CAD build for the part. Positions are in the model's coordinates, mm. Face numbers are marked on the shaded views. A direction names the side the tool comes from. Give positions to 0.01 mm unless a question says otherwise; leave off trailing zeros. Loops run counter-clockwise (first coordinate to the right, second up) from the corner with the lowest first, then second, coordinate; pieces in that order, holes last.
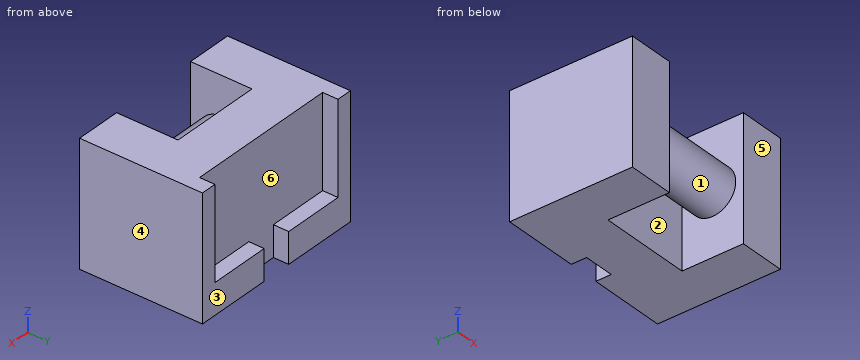
```python
from build123d import *

# Parameters (mm, degrees)
SKETCH2_W           = 76.2
SKETCH2_H           = 25.4
BOSS_EXTRUDE1_DEPTH = 50.8
SKETCH3_W           = 19.05
SKETCH3_H           = 50.8
BOSS_EXTRUDE2_DEPTH = 25.4
SKETCH4_R           = 9.525
BOSS_EXTRUDE3_DEPTH = 50.8
SKETCH7_W           = 12.6492
SKETCH7_H           = 12.7254
CUT_EXTRUDE1_DEPTH  = 6.35


with BuildPart() as part:
    # Sketch2 → Boss-Extrude1 (new body)
    with BuildSketch(Plane.XY):
        with Locations((30.119125683, -4.19863388)):
            Rectangle(SKETCH2_W, SKETCH2_H)
    extrude(amount=BOSS_EXTRUDE1_DEPTH)

    # Sketch3 → Boss-Extrude2 (add)
    with BuildSketch(Plane.XZ.offset(16.89863388)):
        with Locations((1.544125683, 25.4)):
            Rectangle(SKETCH3_W, SKETCH3_H)
        with Locations((58.694125683, 25.4)):
            Rectangle(SKETCH3_W, SKETCH3_H)
    extrude(amount=BOSS_EXTRUDE2_DEPTH)

    # Sketch4 → Boss-Extrude3 (add)
    with BuildSketch(Plane(origin=(11.069125683, 0, 0), x_dir=(0, 0, -1), z_dir=(1, 0, 0))):
        with Locations(Location((-25.4, -29.59863388, 0), (0, 0, 180))):
            Circle(SKETCH4_R)
    extrude(amount=BOSS_EXTRUDE3_DEPTH)

    # Sketch7 → Cut-Extrude1 (cut)
    with BuildSketch(Plane(origin=(0, 8.50136612, 0), x_dir=(1, 0, 0), z_dir=(0, 1, 0))):
        Polygon((-1.610554317, -12.7254), (-1.610554317, -50.8), (61.798005683, -50.8), (61.798005683, -12.7254), (36.418325683, -12.7254), (23.769125683, -12.7254), align=None)
        with Locations((30.093725683, -6.3627)):
            Rectangle(SKETCH7_W, SKETCH7_H)
    extrude(amount=-CUT_EXTRUDE1_DEPTH, mode=Mode.SUBTRACT)


solid = part.part
```
1. Saw through at D-D, the plane y = -21.5. List the corners of the cut face in (x, z), and give its area (3 significant figures).
Responses:
outline: (-7.98, 0) - (11.07, 0) - (11.07, 20.39) - (49.17, 20.39) - (49.17, 0) - (68.22, 0) - (68.22, 50.8) - (49.17, 50.8) - (49.17, 30.41) - (11.07, 30.41) - (11.07, 50.8) - (-7.98, 50.8) - close
area: 2,320 mm2
2. Tool access for the marked faces 1, 2 and 3: list every direction of +Z, -Z, +X, -X, +Y, -Y with a clear straight run to the whole face (end or side of a thin tool).
Responses:
face 1: none
face 2: +Z, -Z
face 3: +Z, -Z, +X, -X, +Y
3. Saw through at A-A, the plane x = 41. List the corners of the cut face in (y, z) (3 decimals).
Responses:
outline: circle Ø19.05 at (-29.599, 25.4); (-16.899, 0) - (8.501, 0) - (8.501, 12.725) - (2.151, 12.725) - (2.151, 50.8) - (-16.899, 50.8) - close
4. Drop a flat-ended pin along its axis: pin 1 (7 mm diameter, centred on x = 5, y = 6.5, fed in from +Z). Give the stop position or say it passes through.
Responses:
pin 1: stops at z = 12.73
5. Probe line 1 along X through (y, z) = (-18.5, 26.5); line 2 along Y through (x, z) = (13, 39); line 3 along Y through (x, z) = (25.5, 17). List the from-to ranges inside material, lowest first.
Responses:
line 1: x = -7.98 to 11.07, 49.17 to 68.22
line 2: y = -16.9 to 2.15
line 3: y = -34.09 to -25.11, -16.9 to 2.15
6. Saw through at B-B, the plane z = 25.4. List the corners of the cut face in (x, y).
Responses:
outline: (-7.98, -42.3) - (11.07, -42.3) - (11.07, -39.12) - (49.17, -39.12) - (49.17, -42.3) - (68.22, -42.3) - (68.22, 8.5) - (61.8, 8.5) - (61.8, 2.15) - (-1.61, 2.15) - (-1.61, 8.5) - (-7.98, 8.5) - close; hole (11.07, -20.07) - (49.17, -20.07) - (49.17, -16.9) - (11.07, -16.9) - close
7. Pull direction X, two halves, no side cores. Call the marked faces 4, 5 and 6: released by +X, released by -X, zero draft, split by the parting line, or undercut.
Responses:
face 4: released by +X
face 5: zero draft
face 6: undercut
8. Saw through at C-C, the plane z = 40.5. List the corners of the cut face in (x, y).
Responses:
outline: (-7.98, -42.3) - (11.07, -42.3) - (11.07, -16.9) - (49.17, -16.9) - (49.17, -42.3) - (68.22, -42.3) - (68.22, 8.5) - (61.8, 8.5) - (61.8, 2.15) - (-1.61, 2.15) - (-1.61, 8.5) - (-7.98, 8.5) - close
